For this review, use the dimensioned drawing (mm, ordinates from the lowest corner) and the shaded views. Coordinates: 2 decimals unless noted, no trailing zeros. Loops run counter-clockwise (first coordinate to the right, second up) from the corner with the lowest first, then second, coordinate; pieces in that order, holes last. Notation, with made-up numbers: M 77.5,40 L 107.5,40 A16 cw 107.5,66 Z; hole C 33,69 d6. An arc over 180 degrees is marked long. One line per item, written item: value.
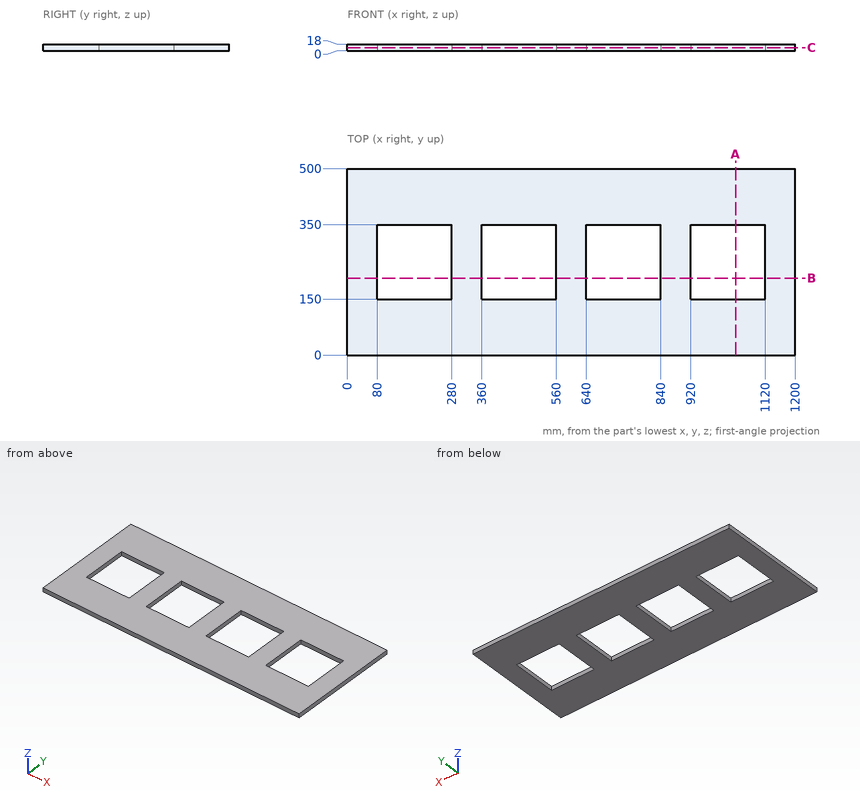
(1) To check wall thickness, follow L1, parallel to X at y = 337, z = 12; L2, parallel to Y at x = 781, z = 5. State the ranges of each line that lie inside material, in increasing order. Write a range as [from, to].
Checks:
L1: [0, 80], [280, 360], [560, 640], [840, 920], [1120, 1200]
L2: [0, 150], [350, 500]
(2) Add section B-B on y = 206.5. State the section outline as (x, z) points, then the cut area to 3 significant figures.
Checks:
outline: M 0,0 L 80,0 L 80,18 L 0,18 Z; M 280,0 L 360,0 L 360,18 L 280,18 Z; M 560,0 L 640,0 L 640,18 L 560,18 Z; M 840,0 L 920,0 L 920,18 L 840,18 Z; M 1120,0 L 1200,0 L 1200,18 L 1120,18 Z
area: 7,200 mm^2
(3) Add section C-C on z = 8.5. State the section outline as (x, y) points, then the cut area to 3 significant figures.
Checks:
outline: M 0,0 L 1200,0 L 1200,500 L 0,500 Z; hole M 80,150 L 280,150 L 280,350 L 80,350 Z; hole M 360,150 L 560,150 L 560,350 L 360,350 Z; hole M 640,150 L 840,150 L 840,350 L 640,350 Z; hole M 920,150 L 1120,150 L 1120,350 L 920,350 Z
area: 440,000 mm^2
(4) Add section A-A on x = 1040.5. State the section outline as (y, z) points, then the cut area to 3 significant figures.
Checks:
outline: M 0,0 L 150,0 L 150,18 L 0,18 Z; M 350,0 L 500,0 L 500,18 L 350,18 Z
area: 5,400 mm^2
